For this review, take the finished solid that the model builds, in its own axes (mm). Face numbers are marked on the shaded views. Give positions to 0.01 mm unless a question says otherwise; leave off trailing zeros. Loops run counter-clockwise (first coordinate to the right, second up) from the corner with the lowest first, then second, coordinate; pieces in that order, holes last.
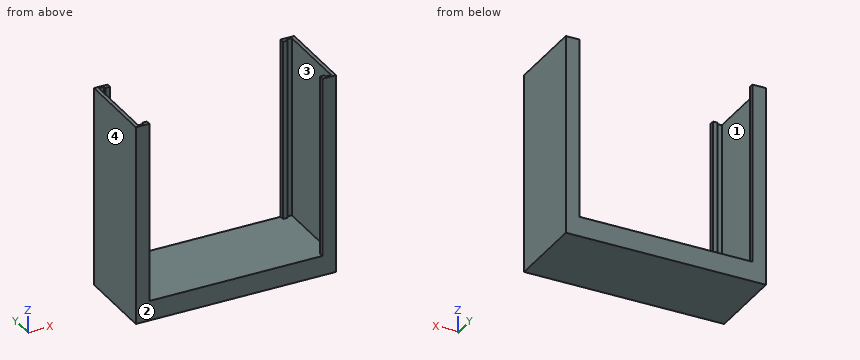
```python
from build123d import *

# Parameters (mm, degrees)
F0_W     = 112.776
F0_H     = 44.704
F1_DEPTH = 11.176
F3_DEPTH = 101.6


with BuildPart() as f1:
    # F0 (on Top) → F1 (new body)
    with BuildSketch(Plane.XY):
        with Locations((-56.388, -22.352)):
            Rectangle(F0_W, F0_H)
    extrude(amount=F1_DEPTH)

    # F2 (on face) → F3 (join)
    with BuildSketch(Plane.XY.offset(11.176)):
        Polygon((0, -44.704), (0, -22.352), (0, 0), (-7.62, 0), (-7.62, -2.54), (-5.08, -2.54), (-5.08, -1.27), (-2.032, -1.27), (-2.032, -22.352), (-2.032, -43.434), (-5.08, -43.434), (-5.08, -42.164), (-7.62, -42.164), (-7.62, -44.704), align=None)
        Polygon((-105.156, -2.54), (-105.156, 0), (-112.776, 0), (-112.776, -22.352), (-112.776, -44.704), (-105.156, -44.704), (-105.156, -42.164), (-107.696, -42.164), (-107.696, -43.434), (-110.744, -43.434), (-110.744, -22.352), (-110.744, -1.27), (-107.696, -1.27), (-107.696, -2.54), align=None)
    extrude(amount=F3_DEPTH)


solid = f1.part
```
Q1. Consider section B-B on y = -23. Give the boundary of the cut face in (x, z).
Answers:
outline: (-112.78, 0) - (0, 0) - (0, 112.78) - (-2.03, 112.78) - (-2.03, 11.18) - (-110.74, 11.18) - (-110.74, 112.78) - (-112.78, 112.78) - close
Q2. Consider section C-C on x = -78.5. Give the boundary of the cut face in (y, z), plus the area to 3 significant figures.
Answers:
outline: (-44.7, 0) - (0, 0) - (0, 11.18) - (-44.7, 11.18) - close
area: 500 mm2
Q3. For probe 1 along Y at (x, z) = (-106, 49); probe 2 along X at (y, z) = (-39.5, 39.5); probe 3 along Z at (x, y) = (-103, -27), list the stretches that pass through material, from the lowest coordinate up.
Answers:
probe 1: y = -44.7 to -42.16, -2.54 to 0
probe 2: x = -112.78 to -110.74, -2.03 to 0
probe 3: z = 0 to 11.18
Q4. Mouldability with a two-part tool opening along Y and no side actions: class the marked faces 1, 2, 3 and 4 as +Y half, -Y half, draft (parallel to the pull), parting line (faces both ways), or undercut.
Answers:
face 1: undercut
face 2: -Y half
face 3: undercut
face 4: draft
Q5. Consider section A-A on z = 95.5. Give the boundary of the cut face in (x, y), plus the area to 3 significant figures.
Answers:
outline: (-112.78, -44.7) - (-105.16, -44.7) - (-105.16, -42.16) - (-107.7, -42.16) - (-107.7, -43.43) - (-110.74, -43.43) - (-110.74, -1.27) - (-107.7, -1.27) - (-107.7, -2.54) - (-105.16, -2.54) - (-105.16, 0) - (-112.78, 0) - close; (-7.62, -44.7) - (0, -44.7) - (0, 0) - (-7.62, 0) - (-7.62, -2.54) - (-5.08, -2.54) - (-5.08, -1.27) - (-2.03, -1.27) - (-2.03, -43.43) - (-5.08, -43.43) - (-5.08, -42.16) - (-7.62, -42.16) - close
area: 223 mm2
Q6. For pin 1 Ø12 at (x, y) = (-18.5, -25) entering from +Z, flat-tipped, find the tip position at first contact; note if it passes through.
Answers:
pin 1: stops at z = 11.18
